Source: CAD feature listing. Evaluate the final solid. Frame: model axes, mm. Give positions to 0.01 mm unless a question says otherwise; leave off trailing zeros. Loops run counter-clockwise (first coordinate to the right, second up) from the corner with the lowest first, then second, coordinate; pieces in that order, holes last. Notation, with made-up numbers: M 43.25,13 L 84.25,13 A17 ccw 84.25,23 Z; hole C -5,-20.5 d8. An arc over 180 degrees is marked long. Answer in a Markdown table with one row per item.
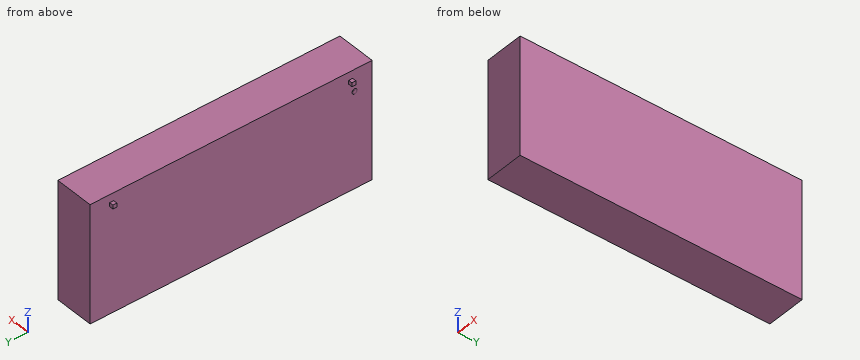
```python
from build123d import *

# Parameters (mm, degrees)
F0_W     = 254
F0_H     = 762
F1_DEPTH = 1828.8
F2_W     = 25.4
F2_H     = 25.4
F3_DEPTH = 25.4
F4_R     = 16.4732072573
F5_DEPTH = 2.54


# Not quite as in the source:
# - a fillet or chamfer that OpenCascade refuses, or shapes differently, is made with other operations: its cross-section is extruded or revolved along the edge and cut away or added


with BuildPart() as f1:
    # F0 (on Front) → F1 (new body)
    with BuildSketch(Plane.XZ):
        Rectangle(F0_W, F0_H)
    extrude(amount=F1_DEPTH)

    # F2 (on face) → F3 (join)
    with BuildSketch(Plane(origin=(-127, 0, 0), x_dir=(0, -1, 0), z_dir=(-1, 0, 0))):
        with Locations((1689.1, 317.5)):
            Rectangle(F2_W, F2_H)
        with Locations((139.7, 317.5)):
            Rectangle(F2_W, F2_H)
    extrude(amount=F3_DEPTH)

    # F4 (on face) → F5 (join)
    with BuildSketch(Plane(origin=(-127, 0, 0), x_dir=(0, -1, 0), z_dir=(-1, 0, 0))):
        with Locations((1714.5154476166, 240.1719689369)):
            Circle(F4_R)
    extrude(amount=F5_DEPTH)

    # F6: fillet of radius 5.08 on 1 edges, made by hand

    # F6_s1 → F6_t2 (revolve, cut)
    with BuildSketch(Plane.XY.offset(240.1719689369)):
        with BuildLine():
            ThreePointArc((-127, -1730.9886548739), (-128.8594090512, -1729.1292458227), (-129.54, -1726.5892458227))
            Line((-129.54, -1726.5892458227), (-129.54, -1730.9886548739))
            Line((-129.54, -1730.9886548739), (-127, -1730.9886548739))
        make_face()
    revolve(axis=Axis((-129.54, -1714.5154476166, 240.1719689369), (-1, 0, 0)), mode=Mode.SUBTRACT)


solid = f1.part
```
Q1. Ray query, probe 1 along X at (y, z) = (-1465.5, -68.5). Return the intervals inside material, ascending. Write a range as from..to.
Values follow:
| item | result |
|---|---|
| probe 1 | -127..127 |
Q2. Contact query for flat-ended pins moving along their axis: pin 1 Ø19.5 at (y, z) = (-1715.5, 244.5) entering from -X; pin 2 Ø7.5 at (x, z) = (-139.5, 318.5) entering from -Y; pin 3 Ø7.5 at (x, y) = (-145, -138.5) entering from -Z. Output: stop coordinate, or through.
Values follow:
| item | result |
|---|---|
| pin 1 | x = -129.54 |
| pin 2 | y = -1701.8 |
| pin 3 | z = 304.8 |
Q3. Section query A-A (y = -1163.5). Output: boundary loops of the cut face in (x, z).
Values follow:
| item | result |
|---|---|
| outline | M -127,-381 L 127,-381 L 127,381 L -127,381 Z |
Q4. Section query B-B (z = 96.5). Output: boundary loops of the cut face in (x, y).
Values follow:
| item | result |
|---|---|
| outline | M -127,-1828.8 L 127,-1828.8 L 127,0 L -127,0 Z |
